The listing builds one solid part. Answer for the finished solid, in the listing's coordinates (mm). A direction names the side the tool comes from. Give positions to 0.01 mm unless a question says otherwise; leave off trailing zeros. Loops run counter-clockwise (first coordinate to the right, second up) from the corner with the lowest first, then second, coordinate; pieces in that order, holes last. Notation, with made-up numbers: M 29,21 L 52,21 A19 ccw 52,55 Z; hole C 33,69 d8. An arc over 180 degrees is marked long. Use one line per item in the form item = value. Start each with the question number.
1. Each of these flat-tipped pins is pushed along its axis until it touches: pin 1 Ø5 at (y, z) = (0, 19.05) entering from +X; pin 2 Ø6.5 at (x, y) = (-9.5, -0.5) entering from +Z; pin 3 Ø1.5 at (y, z) = (-3, 9) entering from +X. Where does it stop, or does it pass through?
2. Straight lines are drawn through the part: line 1 (X direction, y = 1, z = 22.75); line 2 (Y direction, x = -6.35, z = 0.8) (3 decimals); line 3 (Z direction, x = -11.75, y = -2). For each, find the intervals that lie inside material, in ascending order. Write a range as from..to.
3. The part is cut by section B-B (x = -6.35). Write down the section's boundary in (y, z) (3 decimals).
4. The mould has two halves that part along Y. Classify faces 1 (the face through (-24, -6.35, 7)), 2 (the face through (-11, 0, 0)), 3 (the face through (-24.62, 0.69, 15.95)), 4 (the face through (-3.32, 0.95, 0.81)): released by +Y, released by -Y, zero draft, split by the parting line, or undercut.
5. For faces 5 (the face through (-24.49, -0.09, 0.95)), 6 (the face through (-10, 0, 1.6)), determine the directions among +Z, -Z, +X, -X, +Y, -Y from which every point of the face is accessible in a straight line to the end or side of a thin tool.
6. The part is cut by section C-C (y = 0). Give the number of separate pieces and of enclosed holes in the cut face, and give its area (3 significant figures).
from build123d import *

# Parameters (mm, degrees)
F1_DEPTH = 6.35
F2_R     = 3.175
F3_DEPTH = 5.08
F4_R     = 3.175
F5_DEPTH = 5.08


with BuildPart() as f1:
    # F0 (on Front) → F1 (new body, symmetric)
    with BuildSketch(Plane.XZ):
        with BuildLine():
            Line((-22.225, 0), (0, 0))
            Line((0, 0), (0, 1.6002))
            Line((0, 1.6002), (-20.6375, 1.6002))
            ThreePointArc((-20.6375, 1.6002), (-22.882564, 2.530136), (-23.8125, 4.7752))
            Line((-23.8125, 4.7752), (-23.8125, 25.4))
            Line((-23.8125, 25.4), (-25.4, 25.4))
            Line((-25.4, 25.4), (-25.4, 3.175))
            ThreePointArc((-25.4, 3.175), (-24.470064, 0.929936), (-22.225, 0))
        make_face()
    extrude(amount=F1_DEPTH, both=True)

    # F2 (on face) → F3 (cut)
    with BuildSketch(Plane(origin=(-25.4, 0, 0), x_dir=(0, -1, 0), z_dir=(-1, 0, 0))):
        with Locations((0, 19.05)):
            Circle(F2_R)
    extrude(amount=-F3_DEPTH, mode=Mode.SUBTRACT)

    # F4 (on face) → F5 (cut)
    with BuildSketch(Plane.XY.offset(1.6002)):
        with Locations((-6.35, 0)):
            Circle(F4_R)
    extrude(amount=-F5_DEPTH, mode=Mode.SUBTRACT)


solid = f1.part
Derived:
q1.pin_1 = through
q1.pin_2 = 1.6
q1.pin_3 = -23.81
q2.line_1 = -25.4..-23.81
q2.line_2 = -6.35..-3.175, 3.175..6.35
q2.line_3 = 0..1.6
q3.outline = M -6.35,0 L -3.175,0 L -3.175,1.6 L -6.35,1.6 Z; M 3.175,0 L 6.35,0 L 6.35,1.6 L 3.175,1.6 Z
q4.face_1 = released by -Y
q4.face_2 = zero draft
q4.face_3 = undercut
q4.face_4 = undercut
q5.face_5 = -Z, -X, +Y, -Y
q5.face_6 = +Z, +X, +Y, -Y
q6.separate_pieces = 3
q6.enclosed_holes = 0
q6.area = 58.2 mm2
